Design review of the part built by this model. Coordinates are the model's own, in mm. A direction names the side the tool comes from. Coordinates: 2 decimals unless noted, no trailing zeros. Write each loop counter-clockwise with the first axis right and the second up, starting at its lowest first coordinate (ties: lowest second). Pieces come first, ordered by that corner, then holes. Notation, with made-up numbers: M 79,-8 L 115,-8 A35 cw 115,28 Z; hole C -34,-12.5 d5. An arc over 180 degrees is marked long. One line per question, with ' | ' between items.
from build123d import *

# Parameters (mm, degrees)
SKETCH1_R            = 1.7
BOSS_EXTRUDE1_DEPTH  = 2.5
SKETCH1_6_W          = 2.5
SKETCH1_6_H          = 3.9
SKETCH1_6_H_2        = 7.5
BOSS_EXTRUDE3_DEPTH  = 15
BOSS_EXTRUDE8_DEPTH  = 20
BOSS_EXTRUDE9_DEPTH  = 6.5
SKETCH6_9_W          = 23.02
SKETCH6_9_H          = 31.09
SKETCH6_9_W_2        = 18.02
SKETCH6_9_H_2        = 26.09
BOSS_EXTRUDE13_DEPTH = 6.28
SKETCH7_W            = 9.25
SKETCH7_H            = 9.25
BOSS_EXTRUDE14_DEPTH = 35
SKETCH8_R            = 2.25
CUT_EXTRUDE1_DEPTH   = 6.2
CHAMFER1_SIZE        = 0.5
SKETCH9_W            = 1.37
SKETCH9_H            = 5
BOSS_EXTRUDE15_DEPTH = 2.5
CUT_EXTRUDE2_DEPTH   = 5
SKETCH12_W           = 1.38
SKETCH12_H           = 5
BOSS_EXTRUDE16_DEPTH = 2.5
CUT_EXTRUDE3_DEPTH   = 5
CUT_EXTRUDE4_DEPTH   = 5
SKETCH15_W           = 1.38
SKETCH15_H           = 5
BOSS_EXTRUDE17_DEPTH = 2.5
CUT_EXTRUDE5_DEPTH   = 5
CUT_EXTRUDE6_DEPTH   = 5
CUT_EXTRUDE7_DEPTH   = 5


with BuildPart() as part:
    # Sketch1 → Boss-Extrude1 (new body)
    with BuildSketch(Plane.XY):
        Polygon((-49.525, 42.025), (-49.525, 27.025), (-37.335, 27.025), (-37.335, -27.025), (-49.525, -27.025), (-49.525, -42.025), (-7.345, -42.025), (-7.345, -56.715), (7.345, -56.715), (7.345, -42.025), (49.525, -42.025), (49.525, -27.025), (37.335, -27.025), (37.335, -7.345), (52.025, -7.345), (52.025, 7.345), (37.335, 7.345), (37.335, 27.025), (49.525, 27.025), (49.525, 42.025), (7.345, 42.025), (7.345, 56.715), (-7.345, 56.715), (-7.345, 42.025), align=None)
        with Locations((-42.025, -34.525)):
            Circle(SKETCH1_R, mode=Mode.SUBTRACT)
        with Locations((42.025, -34.525)):
            Circle(SKETCH1_R, mode=Mode.SUBTRACT)
        with Locations((-42.025, 34.525)):
            Circle(SKETCH1_R, mode=Mode.SUBTRACT)
        with Locations((42.025, 34.525)):
            Circle(SKETCH1_R, mode=Mode.SUBTRACT)
    extrude(amount=BOSS_EXTRUDE1_DEPTH)

    # Sketch1<6> → Boss-Extrude3 (add)
    with BuildSketch(Plane.XY):
        Polygon((-34.525, -39.525), (-34.525, -42.025), (-7.345, -42.025), (7.345, -42.025), (34.525, -42.025), (34.525, -39.525), align=None)
        Polygon((-34.525, 39.525), (34.525, 39.525), (34.525, 42.025), (7.345, 42.025), (-7.345, 42.025), (-34.525, 42.025), align=None)
        Polygon((34.835, 27.025), (34.835, -27.025), (37.335, -27.025), (37.335, -7.345), (37.335, 7.345), (37.335, 27.025), align=None)
        with Locations((-36.085, 3.675)):
            Rectangle(SKETCH1_6_W, SKETCH1_6_H)
        Polygon((34.835, 39.525), (34.835, 27.025), (37.335, 27.025), (37.335, 42.025), (34.525, 42.025), (34.525, 39.525), align=None)
        Polygon((34.835, -39.525), (34.525, -39.525), (34.525, -42.025), (37.335, -42.025), (37.335, -27.025), (34.835, -27.025), align=None)
        Polygon((-37.335, -34.525), (-37.335, -42.025), (-34.525, -42.025), (-34.525, -39.525), (-34.835, -39.525), (-34.835, -34.525), align=None)
        Polygon((-37.335, -34.182141508), (-37.335, -34.525), (-34.835, -34.525), (-34.835, -27.025), (-37.335, -27.025), align=None)
        with Locations((-36.085, 30.775)):
            Rectangle(SKETCH1_6_W, SKETCH1_6_H_2)
        Polygon((-37.335, 34.525), (-34.835, 34.525), (-34.835, 39.525), (-34.525, 39.525), (-34.525, 42.025), (-37.335, 42.025), align=None)
    extrude(amount=BOSS_EXTRUDE3_DEPTH)

    # Sketch6 → Boss-Extrude8 (add)
    with BuildSketch(Plane.XY.offset(2.5)):
        Polygon((26.685, 32.145), (-24.955, 32.145), (-27.455, 34.645), (29.185, 34.645), (29.185, 5.505), (-27.455, 5.505), (-24.955, 8.005), (26.685, 8.005), align=None)
    extrude(amount=BOSS_EXTRUDE8_DEPTH)

    # Sketch6<4> → Boss-Extrude9 (add)
    with BuildSketch(Plane.XY.offset(2.5)):
        Polygon((5.985, -0.655), (-29.955, -0.655), (-32.455, 1.845), (8.485, 1.845), (8.485, -34.645), (-32.455, -34.645), (-29.955, -32.145), (5.985, -32.145), align=None)
    extrude(amount=BOSS_EXTRUDE9_DEPTH)

    # Sketch6<9> → Boss-Extrude13 (add)
    with BuildSketch(Plane.XY.offset(2.5)):
        with Locations((21.945, -16.4)):
            Rectangle(SKETCH6_9_W, SKETCH6_9_H)
        with Locations((21.945, -16.4)):
            Rectangle(SKETCH6_9_W_2, SKETCH6_9_H_2, mode=Mode.SUBTRACT)
    extrude(amount=BOSS_EXTRUDE13_DEPTH)

    # Sketch7 → Boss-Extrude14 (add)
    with BuildSketch(Plane.XY.offset(2.5)):
        with Locations((0, 49.37)):
            Rectangle(SKETCH7_W, SKETCH7_H)
        with Locations((44.68, 0)):
            Rectangle(SKETCH7_W, SKETCH7_H)
        with Locations((0, -49.37)):
            Rectangle(SKETCH7_W, SKETCH7_H)
    extrude(amount=BOSS_EXTRUDE14_DEPTH)

    # Sketch8 → Cut-Extrude1 (cut)
    with BuildSketch(Plane.XY.offset(37.5)):
        with Locations((0, -49.37)):
            Circle(SKETCH8_R)
        with Locations((44.68, 0)):
            Circle(SKETCH8_R)
        with Locations((0, 49.37)):
            Circle(SKETCH8_R)
    extrude(amount=-CUT_EXTRUDE1_DEPTH, mode=Mode.SUBTRACT)

    # Chamfer1
    chamfer1_edges = [part.edges().sort_by_distance(p)[0] for p in [
        (-2.25, -49.37, 37.5),
        (42.43, 0, 37.5),
        (-2.25, 49.37, 37.5),
    ]]
    chamfer(chamfer1_edges, length=CHAMFER1_SIZE)

    # Sketch9 → Boss-Extrude15 (add)
    with BuildSketch(Plane.ZY.offset(-26.685)):
        with Locations((21.815, 29.645)):
            Rectangle(SKETCH9_W, SKETCH9_H)
        with Locations((21.815, 10.505)):
            Rectangle(SKETCH9_W, SKETCH9_H)
    extrude(amount=BOSS_EXTRUDE15_DEPTH)

    # Sketch10 → Cut-Extrude2 (cut)
    with BuildSketch(Plane(origin=(0, 27.145, 0), x_dir=(1, 0, 0), z_dir=(0, 1, 0))):
        Polygon((26.435, -21.13), (24.185, -22.5), (24.185, -21.13), align=None)
    extrude(amount=CUT_EXTRUDE2_DEPTH, mode=Mode.SUBTRACT)

    # Sketch12 → Boss-Extrude16 (add)
    with BuildSketch(Plane.ZY.offset(-30.955)):
        with Locations((8.09, -5.855)):
            Rectangle(SKETCH12_W, SKETCH12_H)
        with Locations((8.09, -26.945)):
            Rectangle(SKETCH12_W, SKETCH12_H)
    extrude(amount=BOSS_EXTRUDE16_DEPTH)

    # Sketch13 → Cut-Extrude3 (cut)
    with BuildSketch(Plane.XZ.offset(8.355)):
        Polygon((30.705, 7.4), (28.455, 8.78), (28.455, 7.4), align=None)
    extrude(amount=-CUT_EXTRUDE3_DEPTH, mode=Mode.SUBTRACT)

    # Sketch14 → Cut-Extrude4 (cut)
    with BuildSketch(Plane(origin=(0, -24.445, 0), x_dir=(1, 0, 0), z_dir=(0, 1, 0))):
        Polygon((30.705, -7.4), (28.455, -8.78), (28.455, -7.4), align=None)
    extrude(amount=-CUT_EXTRUDE4_DEPTH, mode=Mode.SUBTRACT)

    # Sketch15 → Boss-Extrude17 (add)
    with BuildSketch(Plane.ZY.offset(-5.985)):
        with Locations((8.31, -3.155)):
            Rectangle(SKETCH15_W, SKETCH15_H)
        with Locations((8.31, -29.645)):
            Rectangle(SKETCH15_W, SKETCH15_H)
    extrude(amount=BOSS_EXTRUDE17_DEPTH)

    # Sketch16 → Cut-Extrude5 (cut)
    with BuildSketch(Plane.XZ.offset(5.655)):
        Polygon((3.485, 9), (3.485, 7.62), (5.735, 7.62), align=None)
    extrude(amount=-CUT_EXTRUDE5_DEPTH, mode=Mode.SUBTRACT)

    # Sketch17 → Cut-Extrude6 (cut)
    with BuildSketch(Plane(origin=(0, -27.145, 0), x_dir=(1, 0, 0), z_dir=(0, 1, 0))):
        Polygon((3.485, -9), (3.485, -7.62), (5.735, -7.62), align=None)
    extrude(amount=-CUT_EXTRUDE6_DEPTH, mode=Mode.SUBTRACT)

    # Sketch18 → Cut-Extrude7 (cut)
    with BuildSketch(Plane(origin=(0, 13.005, 0), x_dir=(1, 0, 0), z_dir=(0, 1, 0))):
        Polygon((24.185, -22.5), (24.185, -21.13), (26.435, -21.13), align=None)
    extrude(amount=-CUT_EXTRUDE7_DEPTH, mode=Mode.SUBTRACT)


solid = part.part
1. Insertion check: pin 1 Ø4 at (x, y) = (28, 22) entering from -Z; pin 2 Ø2.5 at (x, y) = (44.68, 0) entering from +Z; pin 3 Ø2 at (y, z) = (32.5, 1) entering from +X (3 decimals); pin 4 Ø4.5 at (y, z) = (49, 26.5) entering from +X (3 decimals). Each pin has a flat end and moves straight along its axis. Give the tip position at first contact, or say it passes through.
Answer sheet:
pin 1: z = 0 | pin 2: z = 31.3 | pin 3: x = 49.525 | pin 4: x = 4.625
2. Take a section at C-C (x = -23.5). Write out the cut boundary in (y, z) (3 decimals), then the cut area to 3 significant figures.
Answer sheet:
outline: M -42.025,0 L 42.025,0 L 42.025,15 L 39.525,15 L 39.525,2.5 L 34.645,2.5 L 34.645,22.5 L 32.145,22.5 L 32.145,2.5 L 8.005,2.5 L 8.005,22.5 L 5.505,22.5 L 5.505,2.5 L 1.845,2.5 L 1.845,9 L -0.655,9 L -0.655,2.5 L -32.145,2.5 L -32.145,9 L -34.645,9 L -34.645,2.5 L -39.525,2.5 L -39.525,15 L -42.025,15 Z | area: 405 mm^2
3. Tool access review of faces 4 (the face through (-7.345, -49, 1)), 5 (the face through (45, 35, 2.5)), 6 (the face through (-44, 27.025, 1)), 7 (the face through (22, -0.855, 6)), 8 (the face through (0, 53.995, 20)): name each direction out of +Z, -Z, +X, -X, +Y, -Y from which nothing blocks a thin tool from reaching the whole face with its end or side.
Answer sheet:
face 4: +Z, -Z, -X, -Y | face 5: +Z, +X, +Y | face 6: +Z, -Z, -X | face 7: +Z | face 8: +Z, +X, -X, +Y
4. Take a section at A-A (z = 16.5). Write out the cut boundary in (x, y) (3 decimals).
Answer sheet:
outline: M -27.455,5.505 L 29.185,5.505 L 29.185,34.645 L -27.455,34.645 L -24.955,32.145 L 26.685,32.145 L 26.685,8.005 L -24.955,8.005 Z; M -4.625,-53.995 L 4.625,-53.995 L 4.625,-44.745 L -4.625,-44.745 Z; M -4.625,44.745 L 4.625,44.745 L 4.625,53.995 L -4.625,53.995 Z; M 40.055,-4.625 L 49.305,-4.625 L 49.305,4.625 L 40.055,4.625 Z
5. Take a section at B-B (y = 49.37). Write out the cut boundary in (x, z) (3 decimals), then the cut area to 3 significant figures.
Answer sheet:
outline: M -7.345,0 L 7.345,0 L 7.345,2.5 L 4.625,2.5 L 4.625,37.5 L 2.75,37.5 L 2.25,37 L 2.25,31.3 L -2.25,31.3 L -2.25,37 L -2.75,37.5 L -4.625,37.5 L -4.625,2.5 L -7.345,2.5 Z | area: 332 mm^2
6. To check wall thickness, follow line 1 along Y through (x, z) = (-20.5, 8.5) (3 decimals); line 2 along Y through (x, z) = (0, 35) (3 decimals); line 3 along X through (y, z) = (19.5, 3) (3 decimals). State the ranges of each line that lie inside material, in increasing order. Write a range as [from, to].
Answer sheet:
line 1: [-42.025, -39.525], [-34.645, -32.145], [-0.655, 1.845], [5.505, 8.005], [32.145, 34.645], [39.525, 42.025] | line 2: [-53.995, -51.62], [-47.12, -44.745], [44.745, 47.12], [51.62, 53.995] | line 3: [26.685, 29.185], [34.835, 37.335]
7. Take a section at D-D (y = -14). Write out the cut boundary in (x, z) (3 decimals).
Answer sheet:
outline: M -37.335,0 L 37.335,0 L 37.335,15 L 34.835,15 L 34.835,2.5 L 33.455,2.5 L 33.455,8.78 L 30.955,8.78 L 30.955,2.5 L 12.935,2.5 L 12.935,8.78 L 10.435,8.78 L 10.435,2.5 L 8.485,2.5 L 8.485,9 L 5.985,9 L 5.985,2.5 L -37.335,2.5 Z
8. Draft analysis for pull direction X (two halves, no side actions). For faces 1 (the face through (4.625, 49, 20)), 2 (the face through (22, -3.355, 6)), 3 (the face through (0, 44.745, 20)), state which applies: pulls with the +X half, pulls with the -X half, needs draft (parallel to the pull), parting line crosses it, or undercut.
Answer sheet:
face 1: pulls with the +X half | face 2: undercut | face 3: needs draft
